Can you work these out from the drawing? Everything is in mm from the part's minimum corner. Round coordinates to 2 decimals unless told otherwise and drop trailing zeros. Write each loop counter-clockwise with the first axis right and the second up, starting at its lowest first coordinate (ties: lowest second). Pieces come first, ordered by that corner, then holes. Notation, with made-up numbers: (39.5, 45) - (91.5, 45) arc R15 cw to (91.5, 51) - close; hole circle Ø2 at (-27.5, -22.5). An arc over 180 degrees is marked (long way). One line per item, written item: value. Start each with the question number.
(1) I want a section at B-B on x = 30. List the corners of the cut face in (y, z) for me, plus the area to 3 significant figures.
(2) I want a section at A-A on z = 30. List the corners of the cut face in (x, y) for me.
(3) If I drill on L1, parallel to X at y = 2.85, z = 30; L2, parallel to Z at x = 40.5, y = 3.7 (1 decimal); L3, parallel to X at y = 3.05, z = 19 (1 decimal), over which ranges is the centre line in solid material (lowest first)? Write a range as from..to.
(4) I'm going to push flat-ended pins straight in: pin 1 Ø1.9 at (x, z) = (19, 19) entering from +Y; pin 2 Ø1.5 at (x, z) = (15.5, 24) entering from -Y; pin 3 Ø1.5 at (y, z) = (3.5, 47.5) entering from +X. Where does each tip first touch, or does it pass through?
(5) I want a section at C-C on y = 1.85. Give the number of separate pieces and of enclosed holes in the cut face, plus the area to 3 significant figures.
(6) I want a section at D-D on x = 41. List the corners of the cut face in (y, z) for me, plus the area to 3 significant figures.
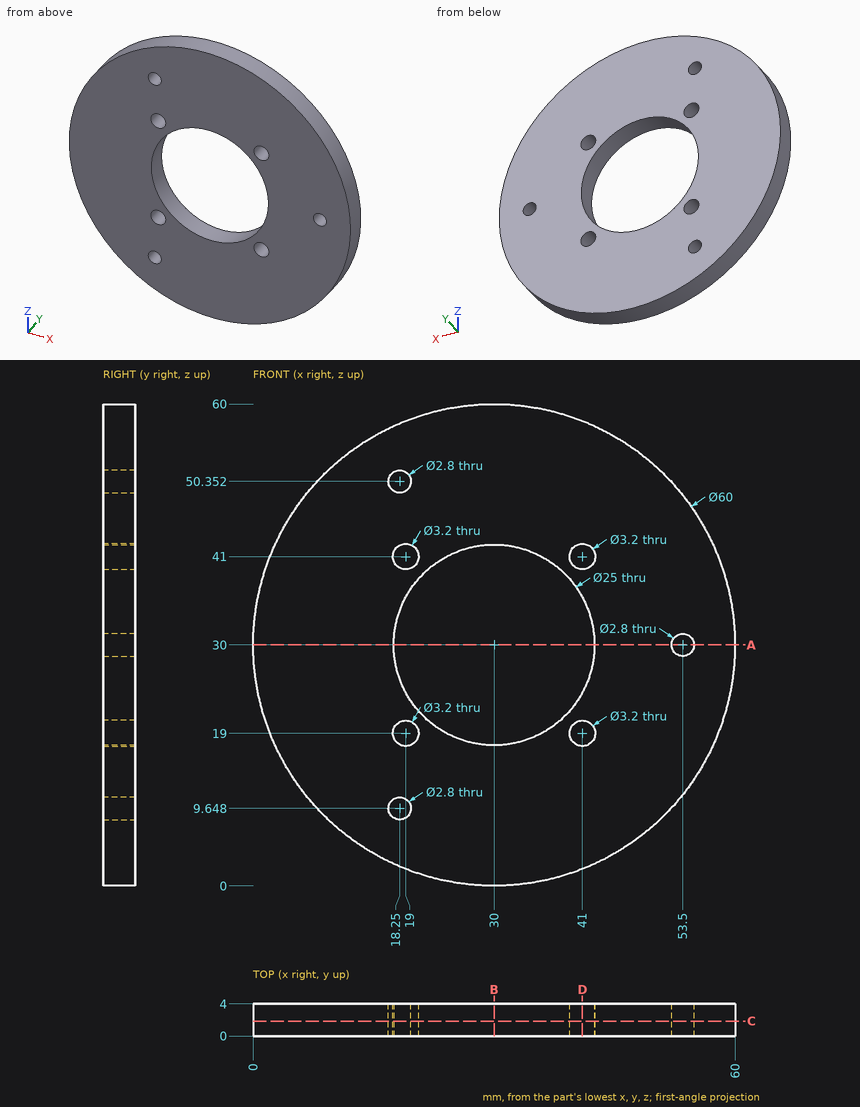
Established:
1. outline: (0, 0) - (4, 0) - (4, 17.5) - (0, 17.5) - close; (0, 42.5) - (4, 42.5) - (4, 60) - (0, 60) - close
1. area: 140 mm2
2. outline: (0, 0) - (17.5, 0) - (17.5, 4) - (0, 4) - close; (42.5, 0) - (52.1, 0) - (52.1, 4) - (42.5, 4) - close; (54.9, 0) - (60, 0) - (60, 4) - (54.9, 4) - close
3. L1: 0..17.5, 42.5..52.1, 54.9..60
3. L2: 1.9..17.5, 20.5..23.2, 36.8..39.5, 42.5..58.1
3. L3: 2.1..17.4, 20.6..24.1, 35.9..39.4, 42.6..57.9
4. pin 1: through
4. pin 2: y = 0
4. pin 3: x = 54.89
5. separate pieces: 1
5. enclosed holes: 8
5. area: 2,290 mm2
6. outline: (0, 2.09) - (4, 2.09) - (4, 17.4) - (0, 17.4) - close; (0, 20.6) - (4, 20.6) - (4, 24.06) - (0, 24.06) - close; (0, 35.94) - (4, 35.94) - (4, 39.4) - (0, 39.4) - close; (0, 42.6) - (4, 42.6) - (4, 57.91) - (0, 57.91) - close
6. area: 150 mm2
